```python
from build123d import *
from build123d.topology import SkipClean

# Parameters (mm, degrees)
SKETCH1_R           = 50.165
BOSS_EXTRUDE1_DEPTH = 20.32
SKETCH4_W           = 6.858
SKETCH4_H           = 39.37
BOSS_EXTRUDE3_DEPTH = 7.62
BOSS_EXTRUDE4_DEPTH = 30.48
BOSS_EXTRUDE5_DEPTH = 15.24


with BuildPart() as part:
    # Sketch1 → Boss-Extrude1 (new body)
    with BuildSketch(Plane.XY):
        Circle(SKETCH1_R)
        with BuildLine():
            Line((16.764, -19.685), (23.622, -19.685))
            Line((23.622, -19.685), (23.622, 19.685))
            Line((23.622, 19.685), (-23.622, 19.685))
            Line((-23.622, 19.685), (-23.622, -19.685))
            Line((-23.622, -19.685), (-16.764, -19.685))
            ThreePointArc((-16.764, -19.685), (0, -29.98053413), (16.764, -19.685))
        make_face(mode=Mode.SUBTRACT)
    extrude(amount=BOSS_EXTRUDE1_DEPTH)

    # Sketch4 → Boss-Extrude3 (add)
    with BuildSketch(Plane(origin=(0, 0, 0), x_dir=(-1, 0, 0), z_dir=(0, 0, -1))):
        with Locations((-20.193, 0)):
            Rectangle(SKETCH4_W, SKETCH4_H)
        with Locations((20.193, 0)):
            Rectangle(SKETCH4_W, SKETCH4_H)
    extrude(amount=-BOSS_EXTRUDE3_DEPTH)

    # Sketch5 → Boss-Extrude4 (add)
    with BuildSketch(Plane.XY.offset(20.32)):
        with BuildLine():
            ThreePointArc((-18.288, -21.463), (0, -31.496), (18.288, -21.463))
            Line((18.288, -21.463), (25.4, -21.463))
            Line((25.4, -21.463), (25.4, 21.463))
            Line((25.4, 21.463), (-25.4, 21.463))
            Line((-25.4, 21.463), (-25.4, -21.463))
            Line((-25.4, -21.463), (-18.288, -21.463))
        make_face()
        with BuildLine():
            Line((-16.764, -19.685), (-23.622, -19.685))
            Line((-23.622, -19.685), (-23.622, 19.685))
            Line((-23.622, 19.685), (23.622, 19.685))
            Line((23.622, 19.685), (23.622, -19.685))
            Line((23.622, -19.685), (16.764, -19.685))
            ThreePointArc((16.764, -19.685), (0, -29.98053413), (-16.764, -19.685))
        make_face(mode=Mode.SUBTRACT)
    extrude(amount=BOSS_EXTRUDE4_DEPTH)

    # Sketch6 → Boss-Extrude5 (add)
    with BuildSketch(Plane.XY.offset(20.32)):
        with BuildLine():
            Line((47.411991955, 16.389943375), (45.251445486, 15.64305988))
            ThreePointArc((45.251445486, 15.64305988), (47.827461768, 2.220932657), (46.506398035, -11.382160729))
            Line((46.506398035, -11.382160729), (48.726862662, -11.925606068))
            ThreePointArc((48.726862662, -11.925606068), (50.111001056, 2.326971882), (47.411991955, 16.389943375))
        make_face()
    boss_extrude5 = extrude(amount=BOSS_EXTRUDE5_DEPTH)

    # Sketch8 → Ø4.0mm Dowel Hole1 (revolve, cut)
    with BuildSketch(Plane(origin=(50.068129829, 3.116023177, 27.647369776), x_dir=(-0.062115482456496916, 0.9980689689791966, 0), z_dir=(0, 0, 1))):
        Polygon((0, 0), (0, 5.011721238), (2, 3.81), (2, 0.020977491), (2.025, 0), align=None)
    f_4_0mm_dowel_hole1 = revolve(axis=Axis((56.405867782, 3.510456491, 27.647369776), (-0.9980689689791966, -0.06211548245649691, 0)), mode=Mode.SUBTRACT)

    # Mirror1: Boss-Extrude5, Ø4.0mm Dowel Hole1 across plane
    with SkipClean():  # the faces are left unmerged after this step: merging them gives an invalid solid
        add(boss_extrude5.mirror(Plane(origin=(0, 0, 0), x_dir=(0, 0, 1), z_dir=(1, 0, 0))))
        add(f_4_0mm_dowel_hole1.mirror(Plane(origin=(0, 0, 0), x_dir=(0, 0, 1), z_dir=(1, 0, 0))), mode=Mode.SUBTRACT)


solid = part.part
```
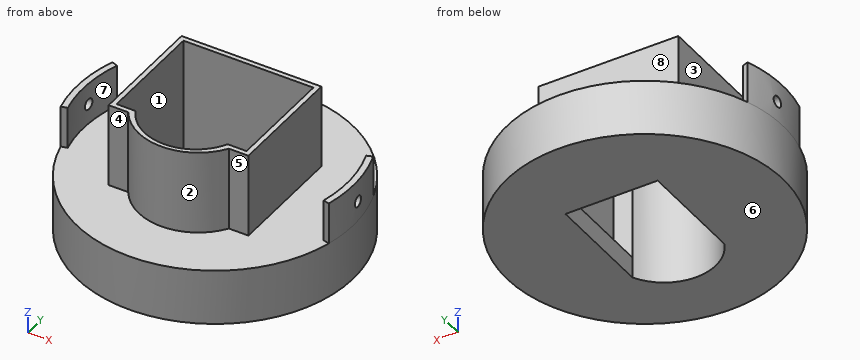
Read the model definition and answer for the solid it produces. Units are mm, in the model's axes. Face numbers are marked on the shaded views. A direction names the side the tool comes from. Give positions to 0.01 mm unless a question says otherwise; leave off trailing zeros. Loops run counter-clockwise (first coordinate to the right, second up) from the corner with the lowest first, then second, coordinate; pieces in that order, holes last.
Item 1: The part is cut by section A-A (x = 0). Write down the section's boundary in (y, z) (3 decimals).
Item 2: Find the intervals of material crossed by line 1 along X through (y, z) = (3, 43.5); line 2 along Z through (x, y) = (21, 42.5); line 3 along Y through (x, z) = (20, 34) (3 decimals), in increasing order.
Item 3: For the marked faces 1, 2, 3 and 4, determine the directions among +Z, -Z, +X, -X, +Y, -Y from which every point of the face is accessible in a straight line to the end or side of a thin tool.
Item 4: The part is cut by section C-C (y = -26). Write down the section's boundary in (x, z), and give its area (3 significant figures).
Item 5: The mould has two halves that part along Y. Classify the marked faces 5, 6, 7 and 8: released by +Y, released by -Y, zero draft, split by the parting line, or undercut.
Item 6: Each of these flat-tipped pins is pushed along its axis until it touches: pin 1 Ø1.5 at (x, y) = (47, 8) entering from +Z; pin 2 Ø2 at (x, z) = (20.5, 21) entering from +Y; pin 3 Ø24.5 at (y, z) = (-5.5, 39.5) entering from +X (3 decimals). Where does it stop, or does it pass through?
Item 7: The part is cut by section B-B (z = 45.5). Write down the section's boundary in (x, y) (3 decimals).
Item 8: The part is cut by section D-D (z = 12.5). Write down the section's boundary in (x, y) (3 decimals).
Taken from the geometry:
1. outline: (-50.165, 0) - (-29.981, 0) - (-29.981, 50.8) - (-31.496, 50.8) - (-31.496, 20.32) - (-50.165, 20.32) - close; (19.685, 0) - (50.165, 0) - (50.165, 20.32) - (21.463, 20.32) - (21.463, 50.8) - (19.685, 50.8) - close
2. line 1: x = -25.4 to -23.62, 23.62 to 25.4
2. line 2: z = 0 to 20.32
2. line 3: y = -21.463 to -19.685, 19.685 to 21.463
3. face 1: +Z
3. face 2: +Z, -Y
3. face 3: +Z, +Y, -Y
3. face 4: +Z, -X, -Y
4. outline: (-42.9, 0) - (-11.57, 0) - (-11.57, 50.8) - (-14.43, 50.8) - (-14.43, 20.32) - (-42.9, 20.32) - close; (11.57, 0) - (42.9, 0) - (42.9, 20.32) - (14.43, 20.32) - (14.43, 50.8) - (11.57, 50.8) - close
4. area: 1,450 mm2
5. face 5: released by -Y
5. face 6: zero draft
5. face 7: undercut
5. face 8: released by +Y
6. pin 1: stops at z = 35.56
6. pin 2: stops at y = 46.11
6. pin 3: stops at x = 50.165
7. outline: (-25.4, -21.463) - (-18.288, -21.463) arc R21.684 ccw to (18.288, -21.463) - (25.4, -21.463) - (25.4, 21.463) - (-25.4, 21.463) - close; hole (-23.622, -19.685) - (-16.764, -19.685) arc R18.796 ccw to (16.764, -19.685) - (23.622, -19.685) - (23.622, 19.685) - (-23.622, 19.685) - close
8. outline: circle Ø100.33 at (0, 0); hole (-23.622, -19.685) - (-16.764, -19.685) arc R18.796 ccw to (16.764, -19.685) - (23.622, -19.685) - (23.622, 19.685) - (-23.622, 19.685) - close
